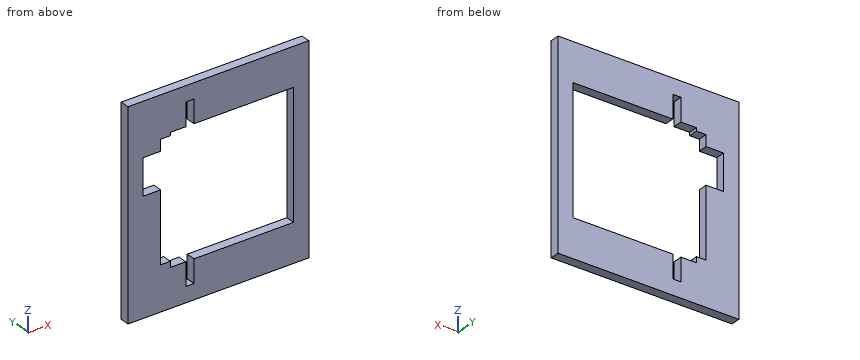
Autodesk Inventor part; units mm, degrees
ref_plane "YZ Plane" through (0, 0, 0) normal (1, 0, 0) x (0, 1, 0)
ref_plane "XZ Plane" through (0, 0, 0) normal (0, 1, 0) x (-1, 0, 0)
ref_plane "XY Plane" through (0, 0, 0) normal (0, 0, 1) x (1, 0, 0)
sketch "Sketch1" plane through (0, 0, 0) normal (0, 1, 0) x (-1, 0, 0)
  line L0 (0, 0) -> (32.08, 0)
  line L1 (39.5, 0) -> (39.5, -1)
  line L2 (39.5, -40.4) -> (34.5, -40.4)
  line L3 (0, -40.4) -> (0, 0)
  line L4 (39.5, -20.2) -> (34.5, -20.2) construction
  line L5 (34.5, 7.45) -> (32.08, 7.45)
  line L6 (32.08, 7.45) -> (32.08, 0)
  line L7 (32.08, -47.85) -> (34.5, -47.85)
  line L8 (34.5, -47.85) -> (34.5, -40.4)
  line L9 (42.6, -1) -> (39.5, -1)
  line L10 (39.5, -1) -> (39.5, -38.55) construction
  line L11 (39.5, -38.55) -> (42.6, -38.55)
  line L12 (42.6, -38.55) -> (42.6, -16.01)
  line L13 (48.25, -4.61) -> (42.6, -4.61)
  line L14 (42.6, -4.61) -> (42.6, -16.01) construction
  line L15 (42.6, -16.01) -> (48.25, -16.01)
  line L16 (48.25, -16.01) -> (48.25, -4.61)
  line L17 (48.25, 7.45) -> (0, 7.45) construction
  line L18 (0, 7.45) -> (0, -47.85) construction
  line L19 (0, -47.85) -> (48.25, -47.85) construction
  line L20 (48.25, -47.85) -> (48.25, 7.45) construction
  line L21 (-5, 12.45) -> (53.25, 12.45)
  line L22 (53.25, 12.45) -> (53.25, -52.85)
  line L23 (53.25, -52.85) -> (-5, -52.85)
  line L24 (-5, -52.85) -> (-5, 12.45)
  line L25 (34.5, 0) -> (39.5, 0)
  line L26 (32.08, 0) -> (34.5, 0) construction
  line L27 (34.5, -40.4) -> (32.08, -40.4) construction
  line L28 (32.08, -40.4) -> (0, -40.4)
  line L29 (39.5, -1) -> (39.5, -38.55) construction
  line L30 (39.5, -38.55) -> (39.5, -40.4)
  line L31 (42.6, -4.61) -> (42.6, -1)
  line L32 (42.6, -16.01) -> (42.6, -4.61) construction
  line L33 (32.08, 0) -> (32.08, -40.4) construction
  line L34 (34.5, 0) -> (34.5, 7.45)
  line L35 (34.5, -40.4) -> (34.5, 0) construction
  line L36 (32.08, -40.4) -> (32.08, -47.85)
  line L37 (34.6, 7.55) -> (31.98, 7.55)
  line L38 (31.98, 7.55) -> (31.98, 0.1)
  line L39 (31.98, 0.1) -> (-0.1, 0.1)
  line L40 (-0.1, 0.1) -> (-0.1, -40.5)
  line L41 (-0.1, -40.5) -> (31.98, -40.5)
  line L42 (31.98, -40.5) -> (31.98, -47.95)
  line L43 (31.98, -47.95) -> (34.6, -47.95)
  line L44 (34.6, -47.95) -> (34.6, -40.5)
  line L45 (34.6, -40.5) -> (39.6, -40.5)
  line L46 (39.6, -40.5) -> (39.6, -38.65)
  line L47 (39.6, -38.65) -> (42.7, -38.65)
  line L48 (42.7, -38.65) -> (42.7, -16.11)
  line L49 (42.7, -16.11) -> (48.35, -16.11)
  line L50 (48.35, -16.11) -> (48.35, -4.51)
  line L51 (48.35, -4.51) -> (42.7, -4.51)
  line L52 (42.7, -4.51) -> (42.7, -0.9)
  line L53 (42.7, -0.9) -> (39.6, -0.9)
  line L54 (39.6, -0.9) -> (39.6, 0.1)
  line L55 (39.6, 0.1) -> (34.6, 0.1)
  line L56 (34.6, 0.1) -> (34.6, 7.55)
  point P0 (41.05, -1)
  point P1 (42.6, -10.31)
  point P2 (33.29, -47.85)
  point P3 (48.25, -10.31)
  point P4 (33.29, 7.45)
  point P5 (0, -20.2)
  dimension "d0" = 39.5
  dimension "d1" = 40.4
  dimension "d2" = 5
  dimension "d3" = 2.42
  dimension "d4" = 55.3
  dimension "d5" = 3.1
  dimension "d6" = 37.55
  dimension "d8" = 5.65
  dimension "d9" = 11.4
  dimension "d10" = 4.61
  dimension "d11" = 5
  dimension "d12" = 0.1
extrude "Extrusion1" add sketch "Sketch1" along normal blind 3 contours L21 L22 L23 L24
properties part number "ft5330m_profile_v2"
Input: part model. Units: mm. Frame: model coordinates. Coordinates: 2 decimals unless noted, no trailing zeros. Loops run counter-clockwise (first coordinate to the right, second up) from the corner with the lowest first, then second, coordinate; pieces in that order, holes last.
Q1. Cut plane B-B (z = -19). Output: boundary loops of the cut face in (x, y).
Q2. Cut plane C-C (x = -22). Output: boundary loops of the cut face in (y, z).
Q3. Material intervals for line 1 (Z direction, x = -22.5, y = 1.95); line 2 (X direction, y = 0.4, z = -18.5); line 3 (X direction, y = 2.3, z = -15), sorted ascending.
Q4. Cut plane A-A (y = 2.25). Output: boundary loops of the cut face in (x, z), then the cut area to 3 significant figures.
Working result:
1. outline: (-53.25, 0) - (-42.7, 0) - (-42.7, 3) - (-53.25, 3) - close; (0.1, 0) - (5, 0) - (5, 3) - (0.1, 3) - close
2. outline: (0, -52.85) - (3, -52.85) - (3, -40.5) - (0, -40.5) - close; (0, 0.1) - (3, 0.1) - (3, 12.45) - (0, 12.45) - close
3. line 1: z = -52.85 to -40.5, 0.1 to 12.45
3. line 2: x = -53.25 to -42.7, 0.1 to 5
3. line 3: x = -53.25 to -48.35, 0.1 to 5
4. outline: (-53.25, -52.85) - (5, -52.85) - (5, 12.45) - (-53.25, 12.45) - close; hole (-48.35, -16.11) - (-42.7, -16.11) - (-42.7, -38.65) - (-39.6, -38.65) - (-39.6, -40.5) - (-34.6, -40.5) - (-34.6, -47.95) - (-31.98, -47.95) - (-31.98, -40.5) - (0.1, -40.5) - (0.1, 0.1) - (-31.98, 0.1) - (-31.98, 7.55) - (-34.6, 7.55) - (-34.6, 0.1) - (-39.6, 0.1) - (-39.6, -0.9) - (-42.7, -0.9) - (-42.7, -4.51) - (-48.35, -4.51) - close
4. area: 1,970 mm2
